Input: part model. Units: mm. Frame: model coordinates. Face numbers are marked on the shaded views. Coordinates: 2 decimals unless noted, no trailing zeros. Write each loop counter-clockwise with the first axis right and the second up, starting at its lowest first coordinate (ties: lowest second). Pieces come first, ordered by that corner, then holes. Notation, with made-up numbers: M 46,-28.5 L 74,-28.5 A24 cw 74,-0.5 Z; hole C 6.25,-4.5 d2. An arc over 180 degrees is marked long. Use CSV: the item, a comma, the result in double quotes.
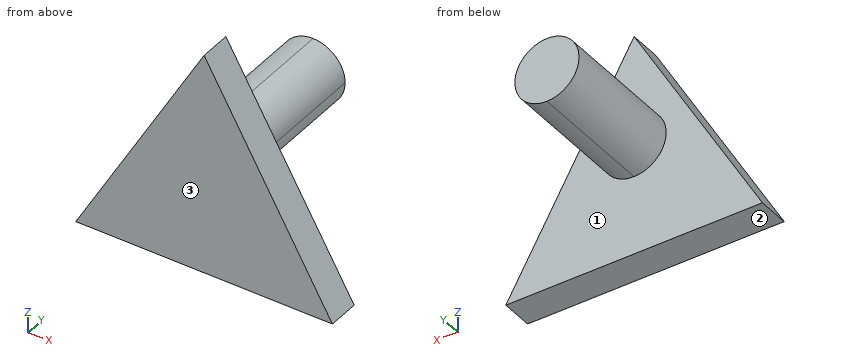
```python
from build123d import *

# Parameters (mm, degrees)
F1_DEPTH = 5
F3_DEPTH = 25


with BuildPart() as f1:
    # F0 (on Front) → F1 (new body)
    with BuildSketch(Plane.XZ):
        Polygon((-20, 0), (0, 0), (20, 0), (0, 34.6410161514), align=None)
    extrude(amount=F1_DEPTH)

    # F2 (on face) → F3 (join)
    with BuildSketch(Plane.XZ.offset(5)):
        with BuildLine():
            Line((0, 22.3205080757), (0, 12.3205080757))
            ThreePointArc((0, 12.3205080757), (3.5355339059, 13.7849741698), (5, 17.3205080757))
            ThreePointArc((5, 17.3205080757), (3.5355339059, 20.8560419816), (0, 22.3205080757))
        make_face()
        with BuildLine():
            ThreePointArc((0, 22.3205080757), (-5, 17.3205080757), (0, 12.3205080757))
            Line((0, 12.3205080757), (0, 22.3205080757))
        make_face()
    extrude(amount=-F3_DEPTH)


solid = f1.part
```
1. Contact query for flat-ended pins moving along their axis: pin 1 Ø3 at (x, z) = (-9, 3.5) entering from +Y; pin 2 Ø12 at (x, y) = (-14, 13) entering from -Z; pin 3 Ø6 at (y, z) = (4.5, 17.5) entering from -X; pin 4 Ø6 at (y, z) = (7, 10.5) entering from +X. Output: stop coordinate, or through.
Resolved:
pin 1,"stops at y = 0"
pin 2,"passes through"
pin 3,"stops at x = -5"
pin 4,"stops at x = 3.23"
2. Material intervals for line 1 (Y direction, x = 9.5, z = 3.5); line 2 (X direction, y = 6.5, z = 17); line 3 (X direction, y = -3.75, z = 8.5), sorted ascending. Write a range as [from, to].
Resolved:
line 1,"y = [-5, 0]"
line 2,"x = [-4.99, 4.99]"
line 3,"x = [-15.09, 15.09]"
3. Mould query, pull axis Y, two halves, no side actions, for the marked faces 1, 2 and 3. Classes: pulls with the +Y half, pulls with the -Y half, needs draft (parallel to the pull), parting line crosses it, or undercut.
Resolved:
face 1,"pulls with the +Y half"
face 2,"needs draft"
face 3,"pulls with the -Y half"
4. Section A-A (z = 14.5). Return loops of the section in (x, y).
Resolved:
outline,"M -11.63,-5 L 11.63,-5 L 11.63,0 L 4.13,0 L 4.13,20 L -4.13,20 L -4.13,0 L -11.63,0 Z"
5. Section B-B (x = 10). Return loops of the section in (y, z), then the cut area to 3 significant figures.
Resolved:
outline,"M -5,0 L 0,0 L 0,17.32 L -5,17.32 Z"
area,"86.6 mm^2"
6. Section C-C (y = 16). Return loops of the section in (x, z).
Resolved:
outline,"C 0,17.32 d10"
7. Section D-D (x = -6). Return loops of the section in (y, z), then the cut area to 3 significant figures.
Resolved:
outline,"M -5,0 L 0,0 L 0,24.25 L -5,24.25 Z"
area,"121 mm^2"
